Input: part model. Units: mm. Frame: model coordinates. A direction names the side the tool comes from. Coordinates: 2 decimals unless noted, no trailing zeros. Write each loop counter-clockwise with the first axis right and the second up, starting at its lowest first coordinate (ties: lowest second). Pieces come first, ordered by that corner, then holes.
from build123d import *

# Parameters (mm, degrees)
EXTRUDE_1_DEPTH     = 410
CUT_EXTRUDE_1_DEPTH = 165
SKETCH_4_R          = 20
SKETCH_4_R_2        = 9.341042427
SKETCH_4_R_3        = 10
EXTRUDE_2_DEPTH     = 30
SKETCH_5_R          = 8.254931616
SKETCH_5_R_2        = 9.226679221
EXTRUDE_3_DEPTH     = 30


with BuildPart() as part:
    # Эскиз2 → Бобышка-Вытянуть1 (new body)
    with BuildSketch(Plane.XY):
        with BuildLine():
            Line((-134, 0), (134, 0))
            Line((134, 0), (134, 211.383370155))
            ThreePointArc((134, 211.383370155), (128.142135624, 225.525505779), (114, 231.383370155))
            Line((114, 231.383370155), (17.613812431, 231.383370155))
            Line((17.613812431, 231.383370155), (17.613812431, 273.795473599))
            Line((17.613812431, 273.795473599), (-17.613812431, 273.795473599))
            Line((-17.613812431, 273.795473599), (-17.613812431, 231.383370155))
            Line((-17.613812431, 231.383370155), (-114, 231.383370155))
            ThreePointArc((-114, 231.383370155), (-128.142135624, 225.525505779), (-134, 211.383370155))
            Line((-134, 211.383370155), (-134, 0))
        make_face()
    extrude(amount=EXTRUDE_1_DEPTH)

    # Эскиз3 → Вырез-Вытянуть1 (cut, symmetric)
    with BuildSketch(Plane(origin=(0, 0, 0), x_dir=(0, 0, -1), z_dir=(1, 0, 0))):
        Polygon((-271.206372328, 273.795473599), (-298.41124171, 231.383370155), (-410.493924083, 231.383370155), (-410.493924083, 334.856445818), (0, 334.856445818), (0, 231.383370155), (-126.94500188, 231.383370155), (-153.338385259, 273.795473599), align=None)
    extrude(amount=CUT_EXTRUDE_1_DEPTH, both=True, mode=Mode.SUBTRACT)

    # Эскиз4 → Бобышка-Вытянуть2 (add)
    with BuildSketch(Plane.XY.offset(410)):
        with Locations((-80, 47.069313646)):
            Circle(SKETCH_4_R)
        with Locations((-40, 47.069313646)):
            Circle(SKETCH_4_R_2)
        with Locations((80.509329497, 47.069313646)):
            Circle(SKETCH_4_R)
        with Locations((-55, 190)):
            Circle(SKETCH_4_R_3)
        with Locations((5, 190)):
            Circle(SKETCH_4_R_3)
    extrude(amount=EXTRUDE_2_DEPTH)

    # Эскиз5 → Бобышка-Вытянуть3 (add)
    with BuildSketch(Plane(origin=(0, 0, 0), x_dir=(-1, 0, 0), z_dir=(0, 0, -1))):
        with Locations((-12.302238961, 29.934052236)):
            Circle(SKETCH_5_R)
        with Locations((-73.813433765, 29.934052236)):
            Circle(SKETCH_5_R_2)
    extrude(amount=EXTRUDE_3_DEPTH)


solid = part.part
Item 1: Section query B-B, the plane z = 356.5. Return loops of the section in (x, y).
Item 2: Section query D-D, the plane z = 171.5. Return loops of the section in (x, y), then the cut area to 3 significant figures.
Item 3: Pull-direction query (X, two-part tool) for faces 1 (the face through (0.247, 252.293, 139.957)), 2 (the face through (2.83, 180.24, 424.79)), 3 (the face through (-17.614, 253, 211)); classes: released by +X, released by -X, zero draft, split by the parting line, or undercut.
Item 4: Material intervals for line 1 (Z direction, x = -74.5, y = 189); line 2 (Y direction, x = 18, z = 247.5); line 3 (X direction, y = 259, z = 184), sorted ascending.
Item 5: Pin query (flat end, axial travel): pin 1 Ø1 at (x, y) = (-81, 193) entering from +Z; pin 2 Ø10 at (x, y) = (-19, 57.5) entering from -Z; pin 3 Ø10 at (x, z) = (-41, 48) entering from +Y. Return the tip coordinate at first contact, or that it passes through.
Item 6: Section query A-A, the plane x = -80. Return loops of the section in (y, z), then the cut area to 3 significant figures.
Item 7: Access query for faces 4 (the face through (17.614, 252, 211)), 5 (the face through (13.38, 38.12, -14.79)), 6 (the face through (-41.22, 56.33, 424.79)). Directions: +Z, -Z, +X, -X, +Y, -Y. A direction counts if a zero-diameter tool reaches every point of the face in a straight line with its end or side. Return the directions, or none.
Item 8: Section query C-C, the plane y = 190. Return loops of the section in (x, z).
The answers:
1. outline: (-134, 0) - (134, 0) - (134, 211.38) arc R20 ccw to (114, 231.38) - (-114, 231.38) arc R20 ccw to (-134, 211.38) - close
2. outline: (-134, 0) - (134, 0) - (134, 211.38) arc R20 ccw to (114, 231.38) - (17.61, 231.38) - (17.61, 273.8) - (-17.61, 273.8) - (-17.61, 231.38) - (-114, 231.38) arc R20 ccw to (-134, 211.38) - close
2. area: 63,300 mm2
3. face 1: zero draft
3. face 2: undercut
3. face 3: released by -X
4. line 1: z = 0 to 410
4. line 2: y = 0 to 231.38
4. line 3: x = -17.61 to 17.61
5. pin 1: stops at z = 410
5. pin 2: stops at z = 0
5. pin 3: stops at y = 231.38
6. outline: (0, 0) - (231.38, 0) - (231.38, 410) - (67.07, 410) - (67.07, 440) - (27.07, 440) - (27.07, 410) - (0, 410) - close
6. area: 96,100 mm2
7. face 4: +Z, -Z, +X, +Y
7. face 5: -Z
7. face 6: +Z
8. outline: (-134, 0) - (134, 0) - (134, 410) - (15, 410) - (15, 440) - (-5, 440) - (-5, 410) - (-45, 410) - (-45, 440) - (-65, 440) - (-65, 410) - (-134, 410) - close
